Geometry check sheet. Reference: the model listing, model coordinates, mm. Face numbers are marked on the shaded views. A direction names the side the tool comes from. Coordinates: 2 decimals unless noted, no trailing zeros. Write each loop counter-clockwise with the first axis right and the second up, starting at its lowest first coordinate (ties: lowest second). Pieces come first, ordered by that corner, then holes. Notation, with made-up numbers: (54, 26) -> (81, 26) arc R15 cw to (81, 45) -> close; hole circle Ø8 at (67.25, 6.5). An arc over 180 degrees is marked (long way). Answer in a Markdown table with one row per item. Add a question column.
1. Mould release check, pull along Z, two halves, no side actions. Record for the marked faces 1, 2, 3 and 4: pulls with the +Z half, pulls with the -Z half, needs draft (parallel to the pull), parting line crosses it, or undercut.
2. Cross-section at D-D on z = 20.5. Record the cut outline in (x, y).
3. Cross-section at C-C on y = 51. Record the cut outline in (x, z), and give its area (3 significant figures).
4. Cross-section at A-A on x = 51.5. Record the cut outline in (y, z).
5. Depth check by flat-ended pin: P1, Ø6, axis at y = 41.5, z = -19, coming from the +X side; P2, Ø6.5, axis at x = 15.5, z = -15, coming from the +Y side; P3, Ø20, axis at x = 12.5, z = 10.5, coming from the -Y side; P4, Ø5, axis at y = 48, z = -8.5, coming from the -X side. Enter the tip coordinate at first touch or a pass-through.
6. Set-up check for the marked faces 5, 6 and 7: record each of +Z, -Z, +X, -X, +Y, -Y from which the full face is reachable in a straight line by a thin tool's end or side.
7. Cross-section at B-B on y = 31. Record the cut outline in (x, z), and give its area (3 significant figures).
8. Scan lines: L1, parallel to Z at x = 15.5, y = 31; L2, parallel to Z at x = 41, y = 25; L3, parallel to Z at x = 15, y = 35. Record each from-to range of solid material in increasing order. Write a range as from..to.
Autodesk Inventor part; units mm, degrees
ref_plane "Work Plane1" through (0, 0, 0) normal (0, 0, 1) x (1, 0, 0)
ref_plane "YZ Plane" through (0, 0, 0) normal (1, 0, 0) x (0, 1, 0)
ref_plane "XZ Plane" through (0, 0, 0) normal (0, 1, 0) x (-1, 0, 0)
sketch "Sketch15" plane through (0, 0, 0) normal (0, 0, 1) x (1, 0, 0)
  circle A0 centre (0, 0) radius 60
  dimension "d88" = 120
extrude "Extrusion7" add sketch "Sketch15" along normal mid plane 60
ref_plane "Work Plane1" through (0, 0, 0) normal (0, 0, 1) x (1, 0, 0)
sketch "Sketch16" plane through (0, 0, 0) normal (0, 0, 1) x (1, 0, 0)
  circle A0 centre (0, 0) radius 60
  circle A1 centre (0, 0) radius 47.5
  dimension "d117" = 95
extrude "Extrusion8" cut sketch "Sketch16" along normal mid plane 18
sketch "Sketch17" plane through (0, 0, 0) normal (0, 0, 1) x (1, 0, 0)
  circle A0 centre (0, 0) radius 60
  line L0 (3, 3) -> (59.925, 3)
  line L1 (3, 3) -> (3, 59.925)
  line L2 (28, 25) -> (0, 25)
  line L3 (0, 25) -> (0, 0)
  line L4 (0, 0) -> (28, 0)
  line L5 (28, 0) -> (28, 25)
  point P0 (28, 3)
  point P1 (3, 25)
  dimension "d118" = 3
  dimension "d119" = 3
  dimension "d120" = 22
  dimension "d121" = 25
extrude "Extrusion9" cut sketch "Sketch17" along normal through all both and the other way through all contours A0 L1 L2 L3 L4 L5 L0 | L5 L4 L3 L2 L1 L0 | L0 L1 L2 L5
sketch "Sketch19" plane through (3, 25, 30) normal (0, -1, 0) x (1, 0, 0)
  line L0 (0, -60) -> (0, 0)
  point P0 (-3, -30)
  point P1 (12.5, -15)
  point P2 (12.5, -45)
  point P3 (0, -30)
  point P4 (12.5, -30)
  point P5 (0, -30)
  dimension "d122" = 30
  dimension "d123" = 15
  dimension "d124" = 12.5
hole "Hole6" at (15.5, 25, 15) at (15.5, 25, -15) at (15.5, 25, 0) direction (0, 1, 0) diameter 4.917 depth 17.1 tip angle 118
fillet "Fillet4" radius 2 2 edges at (3, 59.925, -19.5) (3, 59.925, 19.5)
fillet "Fillet5" radius 5 2 edges at (3, 52.5946, -9) (3, 52.5946, 9)
properties part number "TL20240701-10110CV-029" material "S45C"
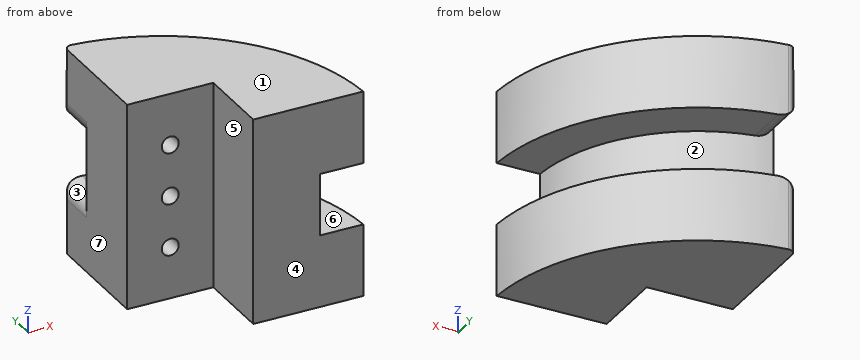
Results found:
| question | item | result |
|---|---|---|
| 1 | face 1 | pulls with the +Z half |
| 1 | face 2 | undercut |
| 1 | face 3 | undercut |
| 1 | face 4 | needs draft |
| 2 | outline | (3, 25) -> (28, 25) -> (28, 3) -> (59.92, 3) arc R60 ccw to (5.17, 59.78) arc R2 ccw to (3, 57.78) -> close |
| 3 | outline | (3, -30) -> (31.61, -30) -> (31.61, -9) -> (8, -9) arc R5 ccw to (3, -14) -> close; (3, 14) arc R5 ccw to (8, 9) -> (31.61, 9) -> (31.61, 30) -> (3, 30) -> close |
| 3 | area | 1,190 mm^2 |
| 4 | outline | (3, -30) -> (30.79, -30) -> (30.79, -9) -> (3, -9) -> close; (3, 9) -> (30.79, 9) -> (30.79, 30) -> (3, 30) -> close |
| 5 | P1 | stops at x = 46.02 |
| 5 | P2 | stops at y = 58.74 |
| 5 | P3 | stops at y = 25 |
| 5 | P4 | stops at x = 3 |
| 6 | face 5 | +Z, -Z, -X, -Y |
| 6 | face 6 | +X, +Y |
| 6 | face 7 | +Z, -Z, -X, +Y, -Y |
| 7 | outline | (3, -30) -> (51.37, -30) -> (51.37, -9) -> (35.99, -9) -> (35.99, 9) -> (51.37, 9) -> (51.37, 30) -> (3, 30) -> close; hole circle Ø4.92 at (15.5, -15); hole circle Ø4.92 at (15.5, 0); hole circle Ø4.92 at (15.5, 15) |
| 7 | area | 2,570 mm^2 |
| 8 | L1 | z = -30..-17.46, -12.54..-2.46, 2.46..12.54, 17.46..30 |
| 8 | L2 | z = -30..-9, 9..30 |
| 8 | L3 | z = -30..-17.41, -12.59..-2.41, 2.41..12.59, 17.41..30 |
